The model under review builds one solid part; all positions refer to its coordinate system, in mm. A direction names the side the tool comes from. Coordinates: 2 decimals unless noted, no trailing zeros. Order: outer loops, then holes, each group sorted by start corner. A loop starts at its lowest first (then second) coordinate and runs counter-clockwise, first axis right, second up. Notation, with made-up numbers: (64.5, -32) -> (78.5, -32) arc R11 cw to (78.5, -16) -> close; hole circle Ø7 at (82.5, 31). An arc over 180 degrees is marked (long way). Use CSV: the item, a comma, the result in double quotes. Start each with the question number.
Autodesk Inventor part; units mm, degrees
ref_plane "Work Plane1" through (0, 15.24, 0) normal (0, 1, 0) x (1, 0, 0)
ref_plane "YZ Plane" through (0, 0, 0) normal (1, 0, 0) x (0, 1, 0)
ref_plane "XZ Plane" through (0, 0, 0) normal (0, 1, 0) x (-1, 0, 0)
sketch "Sketch1" plane through (0, 0, 0) normal (0, 1, 0) x (-1, 0, 0)
  line L0 (31.75, 25.4) -> (-31.75, 25.4)
  line L1 (-31.75, 25.4) -> (-31.75, -25.4)
  line L2 (-31.75, -25.4) -> (31.75, -25.4)
  line L3 (31.75, -25.4) -> (31.75, 25.4)
  line L4 (31.75, 25.4) -> (-31.75, -25.4) construction
  line L5 (-31.75, 25.4) -> (31.75, -25.4) construction
  arc A0 (31.75, -25.4) -> (31.75, 25.4) centre (31.75, 0) ccw
  point P0 (0, 0)
  dimension "d5" = 63.5
  dimension "d6" = 50.8
extrude "Extrusion1" add sketch "Sketch1" against normal blind 8.89
sketch "Sketch2" plane through (0, 0, 0) normal (0, 1, 0) x (1, 0, 0)
  line L0 (31.75, -25.4) -> (31.75, 25.4)
  line L1 (-31.75, -25.4) -> (31.75, -25.4)
  line L2 (31.75, 25.4) -> (-31.75, 25.4)
  arc A0 (-31.75, 25.4) -> (-31.75, -25.4) centre (-31.75, 0) ccw
  line L3 (31.75, 0) -> (16.51, 0)
  line L4 (3.81, -9.525) -> (16.51, -9.525)
  line L5 (16.51, -9.525) -> (16.51, 9.525)
  line L6 (16.51, 9.525) -> (3.81, 9.525)
  line L7 (3.81, 9.525) -> (3.81, -9.525)
  line L8 (3.81, -9.525) -> (16.51, 9.525) construction
  line L9 (16.51, -9.525) -> (3.81, 9.525) construction
  arc A1 (3.81, -9.525) -> (16.51, -9.525) centre (10.16, -9.525) ccw
  arc A2 (16.51, 9.525) -> (3.81, 9.525) centre (10.16, 9.525) ccw
  point P0 (0, 0)
  dimension "d9" = 15.24
  dimension "d10" = 12.7
  dimension "d11" = 19.05
extrude "Extrusion2" cut sketch "Sketch2" against normal blind 8.89 contours L5 L4 L7 L6 | A1 L4 | L6 A2
sketch "Sketch3" plane through (0, 0, 0) normal (0, 1, 0) x (1, 0, 0)
  arc A0 (-31.75, 25.4) -> (-31.75, -25.4) centre (-31.75, 0) ccw
  circle A1 centre (-31.75, 0) radius 25.4
  point P0 (0, 0)
  dimension "d14" = 50.8
ref_plane "Work Plane1" through (0, 15.24, 0) normal (0, 1, 0) x (1, 0, 0)
sketch "Sketch5" plane through (0, 15.24, 0) normal (0, 1, 0) x (1, 0, 0)
  arc A0 (-31.75, 25.4) -> (-31.75, -25.4) centre (-31.75, 0) ccw
  circle A1 centre (-31.75, 0) radius 15.875
  point P0 (0, 0)
  dimension "d20" = 31.75
loft "Loft1" add profiles "Sketch3", "Sketch5"
sketch "Sketch6" plane through (-31.75, 15.24, 0) normal (0, 1, 0) x (1, 0, 0)
  circle A0 centre (0, 0) radius 15.875
  circle A1 centre (0, 0) radius 9.525
  point P0 (31.75, 0)
  dimension "d25" = 19.05
extrude "Extrusion3" cut sketch "Sketch6" against normal blind 50.8 contours A1
properties part number "Coupler for Section"
Q1. Clearance check with flat-ended pins moving along their axes: pin 1 Ø3 at (y, z) = (8.5, 0) entering from -X (3 decimals); pin 2 Ø10 at (y, z) = (-2.5, 1.5) entering from -X; pin 3 Ø5 at (x, y) = (-36.5, 6) entering from +Z; pin 4 Ø12 at (y, z) = (1.5, 20) entering from +X. State where each tip first meets the part, or that it passes through.
Q2. Add section A-A, the plane x = 10.16. State the section outline as (y, z) points (3 decimals).
Q3. Add section C-C, the plane z = 0. State how many separate pieces and enclosed holes the cut face has, then the cut area to 3 significant figures.
Q4. Draft analysis for pull direction X (two halves, no side actions). For faces 1 (the flat face through (-12, -8.89, 0)), 2 (the flat face through (31.75, -4, 0)), 3 (the cylindrical face through (-41.266, 3.344, -0.419)), state which applies: +X half, -X half, draft (parallel to the pull), parting line (faces both ways), or undercut.
Q5. For faces 4 (the cylindrical face through (-57.144, -4.383, -0.559)), 5 (the flat face through (16.51, -4, 0)), list the 3-axis set-ups (+Z, -Z, +X, -X, +Y, -Y) from which the entire face can be reached by the end or side of a thin tool; tool diameter is ignored.
Q6. Add section B-B, the plane y = -1.75. State the section outline as (x, z) points (3 decimals).
Q7. To check wall thickness, follow probe 1 along X at (y, z) = (-3, 0) (3 decimals); probe 2 along Z at (x, y) = (-31.75, -3) (3 decimals); probe 3 along Y at (x, z) = (-6.5, -21). State the ranges of each line that lie inside material, in increasing order.
Answer block:
1,pin 1,"stops at x = -52.775"
1,pin 2,"stops at x = -57.15"
1,pin 3,"stops at z = 22.79"
1,pin 4,"stops at x = 31.75"
2,outline,"(-8.89, -25.4) -> (0, -25.4) -> (0, -15.875) -> (-8.89, -15.875) -> close; (-8.89, 15.875) -> (0, 15.875) -> (0, 25.4) -> (-8.89, 25.4) -> close"
3,separate pieces,"3"
3,enclosed holes,"0"
3,area,"847 mm²"
4,face 1,"draft"
4,face 2,"+X half"
4,face 3,"undercut"
5,face 4,"-X, +Y, -Y"
5,face 5,"+Y, -Y"
6,outline,"(-31.75, -25.4) -> (31.75, -25.4) -> (31.75, 25.4) -> (-31.75, 25.4) arc R25.4 ccw to start; hole circle Ø19.05 at (-31.75, 0); hole (3.81, -9.525) arc R6.35 ccw to (16.51, -9.525) -> (16.51, 9.525) arc R6.35 ccw to (3.81, 9.525) -> close"
7,probe 1,"x = -57.15 to -41.275, -22.225 to 3.81, 16.51 to 31.75"
7,probe 2,"z = -25.4 to -9.525, 9.525 to 25.4"
7,probe 3,"y = -8.89 to 0"
